Verification items for the finished model (mm, model axes). A direction names the side the tool comes from. Round coordinates to 2 decimals unless told otherwise and drop trailing zeros. Order: outer loops, then holes, each group sorted by start corner. A loop starts at its lowest first (then second) coordinate and runs counter-clockwise, first axis right, second up. Notation, with made-up numbers: M 24,61.25 L 38,61.25 A19 cw 38,96.25 Z; hole C 57,84 d9. An arc over 180 degrees is marked long. One line per item, written item: value. Start each with the question number.
from build123d import *

# Parameters (mm, degrees)
SKETCH1_W              = 40
SKETCH1_H              = 40
BODY_DEPTH             = 20
SKETCH2_R              = 0.8
ROTORSIDE_HOLES_DEPTH  = 10
SKETCH3_R              = 0.8
SLIDERSIDE_HOLES_DEPTH = 10
SKETCH4_R              = 6.5
ROTOREXTEND_DEPTH      = 1.6
SKETCH5_R              = 3
ROTOR_DEPTH            = 4
SLIDEREXTEND_START     = 1.6
SKETCH6_R              = 6.5
SLIDEREXTEND_DEPTH     = 1.6
SLIDER_START           = 4
SKETCH7_R              = 3
SLIDER_DEPTH           = 4


with BuildPart() as part:
    # Sketch1 → Body (new body)
    with BuildSketch(Plane(origin=(0, 0, 0), x_dir=(1, 0, 0), z_dir=(0, 1, 0))):
        with Locations((20, 20)):
            Rectangle(SKETCH1_W, SKETCH1_H)
    extrude(amount=BODY_DEPTH)

    # Sketch2 → RotorSide-Holes (cut)
    with BuildSketch(Plane(origin=(0, 20, 0), x_dir=(1, 0, 0), z_dir=(0, 0, -1))):
        with Locations(Location((30.05, 3, 0), (0, 0, 180))):
            Circle(SKETCH2_R)
        with Locations(Location((37.05, 10, 0), (0, 0, 180))):
            Circle(SKETCH2_R)
        with Locations(Location((30.05, 17, 0), (0, 0, 180))):
            Circle(SKETCH2_R)
        with Locations(Location((16.83, 2, 0), (0, 0, 180))):
            Circle(SKETCH2_R)
        with Locations(Location((16.83, 18, 0), (0, 0, 180))):
            Circle(SKETCH2_R)
    extrude(amount=ROTORSIDE_HOLES_DEPTH, mode=Mode.SUBTRACT)

    # Sketch3 → SliderSide-Holes (cut)
    with BuildSketch(Plane(origin=(0, 0, -40), x_dir=(-1, 0, 0), z_dir=(0, 0, -1))):
        with Locations((-37.5, 17.5)):
            Circle(SKETCH3_R)
        with Locations((-37.5, 2.5)):
            Circle(SKETCH3_R)
        with Locations((-22.5, 17.5)):
            Circle(SKETCH3_R)
        with Locations((-22.5, 2.5)):
            Circle(SKETCH3_R)
        with Locations((-2.5, 17.5)):
            Circle(SKETCH3_R)
        with Locations((-2.5, 2.5)):
            Circle(SKETCH3_R)
    extrude(amount=-SLIDERSIDE_HOLES_DEPTH, mode=Mode.SUBTRACT)

    # Sketch4 → RotorExtend (add)
    with BuildSketch(Plane.XY):
        with Locations(Location((10, 10, 0), (0, 0, 180))):
            Circle(SKETCH4_R)
    extrude(amount=ROTOREXTEND_DEPTH)

    # Sketch5 → Rotor (add)
    with BuildSketch(Plane.XY.offset(1.6)):
        with Locations((10, 10)):
            Circle(SKETCH5_R)
    extrude(amount=ROTOR_DEPTH)

    # Sketch6 → SliderExtend (add)
    with BuildSketch(Plane(origin=(0, 0, -40), x_dir=(-1, 0, 0), z_dir=(0, 0, -1)).offset(SLIDEREXTEND_START)):
        with Locations((-10, 10)):
            Circle(SKETCH6_R)
    extrude(amount=-SLIDEREXTEND_DEPTH)

    # Sketch7 → Slider (add)
    with BuildSketch(Plane(origin=(0, 0, -41.6), x_dir=(-1, 0, 0), z_dir=(0, 0, -1)).offset(SLIDER_START)):
        with Locations(Location((-10, 10, 0), (0, 0, 180))):
            Circle(SKETCH7_R)
    extrude(amount=-SLIDER_DEPTH)


solid = part.part
1. Draft check along Y on faces 4 (the face through (10, 10, -45.6)), 5 (the face through (37.5, 2.5, -30)), 6 (the face through (20, 0, -20)). Enter one of: released by +Y, released by -Y, zero draft, split by the parting line, or undercut.
2. Section check C-C (y = 14.75). Record the cut outline in (x, z).
3. Tool access check on faces 1 (the face through (7, 11, 1.6)), 2 (the face through (20, 20, -20)), 3 (the face through (12.86, 9.1, -43.63)). Record the directions out of +Z, -Z, +X, -X, +Y, -Y that give a thin tool (end or side, any length) a straight path to the whole face; none if there is none.
4. Depth check by flat-ended pin: pin 1 (2 mm diameter, centred on x = 12.5, z = -19.5, fed in from -Y); pin 2 (0.5 mm diameter, centred on x = 30, y = 3.5, fed in from +Z); pin 3 (1 mm diameter, centred on x = 16.83, y = 18, fed in from -Z); pin 4 (1 mm diameter, centred on x = 2.5, y = 17.5, fed in from -Z). Enter the tip coordinate at first touch or a pass-through.
5. Section check D-D (x = 8.5). Record the cut outline in (y, z).
6. Section check B-B (y = 11.75). Record the cut outline in (x, z), and give its area (3 significant figures).
7. Section check A-A (x = 30.05). Record the cut outline in (y, z).
8. Scan lines: line 1 along Y through (x, z) = (22.5, -33.5); line 2 along Y through (x, z) = (30.05, -3.5); line 3 along X through (y, z) = (17.25, -38). Record each from-to range of solid material in increasing order.
Geometry check:
1. face 4: zero draft
1. face 5: undercut
1. face 6: released by -Y
2. outline: M 0,-40 L 5.56,-40 L 5.56,-41.6 L 14.44,-41.6 L 14.44,-40 L 40,-40 L 40,0 L 14.44,0 L 14.44,1.6 L 5.56,1.6 L 5.56,0 L 0,0 Z
3. face 1: +Z
3. face 2: +Z, -Z, +X, -X, +Y
3. face 3: -Z
4. pin 1: stops at y = 0
4. pin 2: stops at z = -10
4. pin 3: stops at z = -40
4. pin 4: stops at z = -30
5. outline: M 0,-40 L 3.68,-40 L 3.68,-41.6 L 7.4,-41.6 L 7.4,-45.6 L 12.6,-45.6 L 12.6,-41.6 L 16.32,-41.6 L 16.32,-40 L 20,-40 L 20,0 L 16.32,0 L 16.32,1.6 L 12.6,1.6 L 12.6,5.6 L 7.4,5.6 L 7.4,1.6 L 3.68,1.6 L 3.68,0 L 0,0 Z
6. outline: M 0,-40 L 3.74,-40 L 3.74,-41.6 L 7.56,-41.6 L 7.56,-45.6 L 12.44,-45.6 L 12.44,-41.6 L 16.26,-41.6 L 16.26,-40 L 40,-40 L 40,0 L 16.26,0 L 16.26,1.6 L 12.44,1.6 L 12.44,5.6 L 7.56,5.6 L 7.56,1.6 L 3.74,1.6 L 3.74,0 L 0,0 Z
6. area: 1,680 mm²
7. outline: M 0,-40 L 20,-40 L 20,0 L 17.8,0 L 17.8,-10 L 16.2,-10 L 16.2,0 L 3.8,0 L 3.8,-10 L 2.2,-10 L 2.2,0 L 0,0 Z
8. line 1: y = 0 to 1.7, 3.3 to 16.7, 18.3 to 20
8. line 2: y = 0 to 2.2, 3.8 to 16.2, 17.8 to 20
8. line 3: x = 0 to 1.74, 3.26 to 21.74, 23.26 to 36.74, 38.26 to 40
